Source: CAD feature listing. Evaluate the final solid. Frame: model axes, mm. Coordinates: 2 decimals unless noted, no trailing zeros. Write each loop counter-clockwise with the first axis right and the second up, starting at its lowest first coordinate (ties: lowest second). Pieces come first, ordered by that corner, then holes. Notation, with made-up numbers: M 75.5,68.5 L 107.5,68.5 A27 ccw 107.5,106.5 Z; hole C 81,62 d7. An arc over 180 degrees is marked long. Write item = value, one per line. Start each with the question number.
1. Line query: line 1 along Y through (x, z) = (55, 2.6); line 2 along X through (y, z) = (5, 0.3). Output: solid intervals per line, ascending.
2. Section query C-C (y = 30). Output: boundary loops of the cut face in (x, z), then the cut area to 3 significant figures.
3. Section query B-B (x = 5). Output: boundary loops of the cut face in (y, z), then the cut area to 3 significant figures.
4. Section query A-A (y = 5). Output: boundary loops of the cut face in (x, z).
5. Pin query (flat end, axial travel): pin 1 Ø2 at (x, y) = (28.5, 38) entering from +Z; pin 2 Ø2.5 at (x, y) = (41, 40.5) entering from -Z. Return the tip coordinate at first contact, or that it passes through.
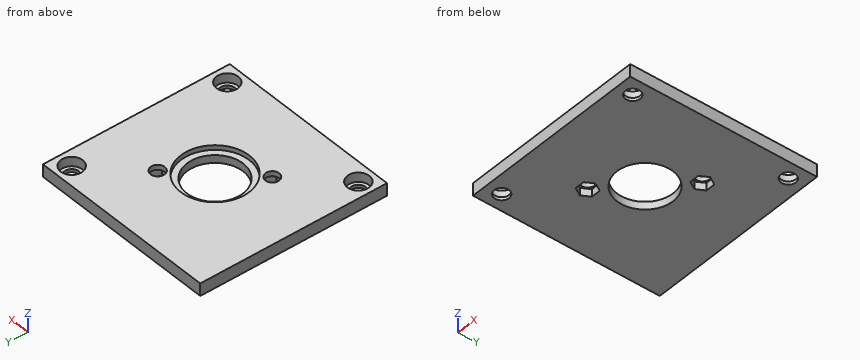
```python
from build123d import *

# Parameters (mm, degrees)
CYLINDER031_R     = 2.25
CYLINDER031_DEPTH = 10
EXTRUDE002_DEPTH  = 2.4
CYLINDER030_R     = 2.2
CYLINDER030_DEPTH = 10
EXTRUDE001_DEPTH  = 2.4
CYLINDER029_R     = 11
CYLINDER029_DEPTH = 10
CYLINDER022_R     = 9
CYLINDER022_DEPTH = 10
CYLINDER024_R     = 3.5
CYLINDER024_DEPTH = 3
CYLINDER023_R     = 2.4
CYLINDER023_DEPTH = 10
CYLINDER026_R     = 3.5
CYLINDER026_DEPTH = 3
CYLINDER025_R     = 2.4
CYLINDER025_DEPTH = 10
CYLINDER028_R     = 3.5
CYLINDER028_DEPTH = 3
CYLINDER027_R     = 2.4
CYLINDER027_DEPTH = 10
BOX005_W          = 60
BOX005_H          = 60
BOX005_DEPTH      = 4


with BuildPart() as cylinder031:
    # Cylinder031 → Cylinder031 (new body)
    with BuildSketch(Plane(origin=(40, 40, 0), x_dir=(1, 0, 0), z_dir=(0, 0, 1))):
        Circle(CYLINDER031_R)
    extrude(amount=CYLINDER031_DEPTH)


with BuildPart() as fusion026:
    # Sketch002 → Extrude002 (new body)
    with BuildSketch(Plane.XY):
        Polygon((-3.005, 0), (-1.5025, -2.602406), (1.5025, -2.602406), (3.005, 0), (1.5025, 2.602406), (-1.5025, 2.602406), align=None)
    extrude(amount=EXTRUDE002_DEPTH)


with BuildPart() as fusion026_1:
    # Extrude002 placement: moved
    add(fusion026.part.moved(Location((40, 40, 0))))

    # Fusion026: union Cylinder031
    add(cylinder031.part)


with BuildPart() as cylinder030:
    # Cylinder030 → Cylinder030 (new body)
    with BuildSketch(Plane(origin=(20, 20, 0), x_dir=(1, 0, 0), z_dir=(0, 0, 1))):
        Circle(CYLINDER030_R)
    extrude(amount=CYLINDER030_DEPTH)


with BuildPart() as compound004:
    # Sketch001 → Extrude001 (new body)
    with BuildSketch(Plane.XY):
        Polygon((-3.005, 0), (-1.5025, -2.602406), (1.5025, -2.602406), (3.005, 0), (1.5025, 2.602406), (-1.5025, 2.602406), align=None)
    extrude(amount=EXTRUDE001_DEPTH)


with BuildPart() as compound004_1:
    # Extrude001 placement: moved
    add(compound004.part.moved(Location((20, 20, 0))))

    # Fusion025: union Cylinder030
    add(cylinder030.part)

    # Compound004: union Fusion026
    add(fusion026_1.part)


with BuildPart() as cylinder029:
    # Cylinder029 → Cylinder029 (new body)
    with BuildSketch(Plane(origin=(30, 30, 2.5), x_dir=(1, 0, 0), z_dir=(0, 0, 1))):
        Circle(CYLINDER029_R)
    extrude(amount=CYLINDER029_DEPTH)


with BuildPart() as cylinder022:
    # Cylinder022 → Cylinder022 (new body)
    with BuildSketch(Plane(origin=(30, 30, 0), x_dir=(1, 0, 0), z_dir=(0, 0, 1))):
        Circle(CYLINDER022_R)
    extrude(amount=CYLINDER022_DEPTH)


with BuildPart() as cylinder024:
    # Cylinder024 → Cylinder024 (new body)
    with BuildSketch(Plane.XY.offset(1)):
        Circle(CYLINDER024_R)
    extrude(amount=CYLINDER024_DEPTH)


with BuildPart() as fusion022:
    # Cylinder023 → Cylinder023 (new body)
    with BuildSketch(Plane.XY):
        Circle(CYLINDER023_R)
    extrude(amount=CYLINDER023_DEPTH)

    # Fusion022: union Cylinder024
    add(cylinder024.part)


with BuildPart() as fusion022_1:
    # Fusion022 placement: moved
    add(fusion022.part.moved(Location((5, 5, 0))))


with BuildPart() as cylinder026:
    # Cylinder026 → Cylinder026 (new body)
    with BuildSketch(Plane.XY.offset(1)):
        Circle(CYLINDER026_R)
    extrude(amount=CYLINDER026_DEPTH)


with BuildPart() as fusion023:
    # Cylinder025 → Cylinder025 (new body)
    with BuildSketch(Plane.XY):
        Circle(CYLINDER025_R)
    extrude(amount=CYLINDER025_DEPTH)

    # Fusion023: union Cylinder026
    add(cylinder026.part)


with BuildPart() as fusion023_1:
    # Fusion023 placement: moved
    add(fusion023.part.moved(Location((55, 5, 0))))


with BuildPart() as cylinder028:
    # Cylinder028 → Cylinder028 (new body)
    with BuildSketch(Plane.XY.offset(1)):
        Circle(CYLINDER028_R)
    extrude(amount=CYLINDER028_DEPTH)


with BuildPart() as compound003:
    # Cylinder027 → Cylinder027 (new body)
    with BuildSketch(Plane.XY):
        Circle(CYLINDER027_R)
    extrude(amount=CYLINDER027_DEPTH)

    # Fusion024: union Cylinder028
    add(cylinder028.part)


with BuildPart() as compound003_1:
    # Fusion024 placement: moved
    add(compound003.part.moved(Location((55, 55, 0))))

    # Compound003: union Fusion022, Fusion023
    add(fusion022_1.part)
    add(fusion023_1.part)


with BuildPart() as obj1:
    # Box005 → Box005 (new body)
    with BuildSketch(Plane.XY):
        with Locations((30, 30)):
            Rectangle(BOX005_W, BOX005_H)
    extrude(amount=BOX005_DEPTH)

    # Cut007: cut Compound003
    add(compound003_1.part, mode=Mode.SUBTRACT)

    # Cut008: cut Cylinder022
    add(cylinder022.part, mode=Mode.SUBTRACT)

    # Cut009: cut Cylinder029
    add(cylinder029.part, mode=Mode.SUBTRACT)

    # Cut010: cut Compound004
    add(compound004_1.part, mode=Mode.SUBTRACT)


solid = obj1.part
```
Results are:
q1.line_1 = 0 to 1.5, 8.5 to 51.5, 58.5 to 60
q1.line_2 = 0 to 2.6, 7.4 to 52.6, 57.4 to 60
q2.outline = M 0,0 L 21,0 L 21,2.5 L 19,2.5 L 19,4 L 0,4 Z; M 39,0 L 60,0 L 60,4 L 41,4 L 41,2.5 L 39,2.5 Z
q2.area = 162 mm^2
q3.outline = M 0,0 L 2.6,0 L 2.6,1 L 1.5,1 L 1.5,4 L 0,4 Z; M 7.4,0 L 60,0 L 60,4 L 8.5,4 L 8.5,1 L 7.4,1 Z
q3.area = 214 mm^2
q4.outline = M 0,0 L 2.6,0 L 2.6,1 L 1.5,1 L 1.5,4 L 0,4 Z; M 7.4,0 L 52.6,0 L 52.6,1 L 51.5,1 L 51.5,4 L 8.5,4 L 8.5,1 L 7.4,1 Z; M 57.4,0 L 60,0 L 60,4 L 58.5,4 L 58.5,1 L 57.4,1 Z
q5.pin_1 = 2.5
q5.pin_2 = 2.4
